Design review of the part built by this model. Coordinates are the model's own, in mm. Face numbers are marked on the shaded views. Round coordinates to 2 decimals unless told otherwise and drop trailing zeros. Order: outer loops, then holes, each group sorted by start corner. A loop starts at its lowest first (then second) coordinate and runs counter-clockwise, first axis right, second up.
from build123d import *

# Parameters (mm, degrees)
BOSS_EXTRUDE1_DEPTH = 6.35
SKETCH2_R           = 1.5875
SKETCH2_W           = 23.495
SKETCH2_H           = 23.495
SKETCH2_R_2         = 8.763
SKETCH2_R_3         = 1.27
SKETCH2_R_4         = 2.159
SKETCH2_R_5         = 2.2225
SKETCH2_R_6         = 31.75
SKETCH2_R_7         = 20.32
SKETCH2_R_8         = 9.525
CUT_EXTRUDE1_DEPTH  = 7.35


with BuildPart() as part:
    # Sketch1 → Boss-Extrude1 (new body)
    with BuildSketch(Plane.XY):
        Polygon((-249.2375, 225.334147625), (249.2375, 225.334147625), (95.25, -225.334147625), (-95.25, -225.334147625), align=None)
    extrude(amount=BOSS_EXTRUDE1_DEPTH)

    # Sketch2 → Cut-Extrude1 (cut, through all)
    with BuildSketch(Plane.XY.offset(6.35)):
        with Locations((-47.625, 15.784147625)):
            Circle(SKETCH2_R)
        with Locations((-47.625, 111.034147625)):
            Circle(SKETCH2_R)
        with Locations((47.625, 15.784147625)):
            Circle(SKETCH2_R)
        with Locations((47.625, 111.034147625)):
            Circle(SKETCH2_R)
        with Locations((0, 174.534147625)):
            Rectangle(SKETCH2_W, SKETCH2_H)
        with Locations((-101.6, 111.034147625)):
            Circle(SKETCH2_R_2)
        with Locations((15, 174.534147625)):
            Circle(SKETCH2_R_3)
        with Locations((-15, 174.534147625)):
            Circle(SKETCH2_R_3)
        with Locations((-40.216666667, -190.409147625)):
            Circle(SKETCH2_R)
        with Locations((-31.75, -203.109147625)):
            Circle(SKETCH2_R)
        with Locations((31.75, -190.409147625)):
            Circle(SKETCH2_R)
        with Locations((40.216666667, -203.109147625)):
            Circle(SKETCH2_R)
        with Locations((-77.7875, -29.409256694)):
            Circle(SKETCH2_R_4)
        with Locations((-23.8125, -29.409256694)):
            Circle(SKETCH2_R_4)
        with Locations((-77.7875, -83.384256694)):
            Circle(SKETCH2_R_4)
        with Locations((-23.8125, -83.384256694)):
            Circle(SKETCH2_R_4)
        with Locations((-83.185, 44.994147625)):
            Circle(SKETCH2_R_5)
        with Locations((-50.8, -56.396756694)):
            Circle(SKETCH2_R_6)
        with Locations((-120.015, 44.994147625)):
            Circle(SKETCH2_R_5)
        with Locations((-120.015, 81.824147625)):
            Circle(SKETCH2_R_5)
        with Locations((-83.185, 81.824147625)):
            Circle(SKETCH2_R_5)
        with Locations((-101.6, 63.409147625)):
            Circle(SKETCH2_R_7)
        with Locations((120.015, 44.994147625)):
            Circle(SKETCH2_R_5)
        with Locations((83.185, 44.994147625)):
            Circle(SKETCH2_R_5)
        with Locations((83.185, 81.824147625)):
            Circle(SKETCH2_R_5)
        with Locations((-83.079166667, 199.934147625)):
            Circle(SKETCH2_R_8)
        with Locations((83.079166667, 199.934147625)):
            Circle(SKETCH2_R_8)
        with Locations((120.015, 81.824147625)):
            Circle(SKETCH2_R_5)
        with Locations((101.6, 63.409147625)):
            Circle(SKETCH2_R_7)
        with Locations((23.8125, -29.409256694)):
            Circle(SKETCH2_R_4)
        with Locations((77.7875, -29.409256694)):
            Circle(SKETCH2_R_4)
        with Locations((23.8125, -83.384256694)):
            Circle(SKETCH2_R_4)
        with Locations((77.7875, -83.384256694)):
            Circle(SKETCH2_R_4)
        with Locations((50.8, -56.396756694)):
            Circle(SKETCH2_R_6)
    extrude(amount=-CUT_EXTRUDE1_DEPTH, mode=Mode.SUBTRACT)


solid = part.part
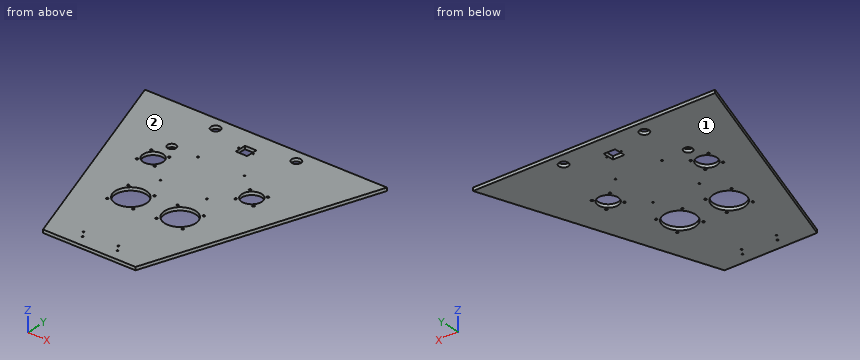
1) Take a section at A-A on y = -64.5. Give the boundary of the cut face in (x, z).
Results:
outline: (-150.2, 0) - (-81.5, 0) - (-81.5, 6.35) - (-150.2, 6.35) - close; (-20.1, 0) - (20.1, 0) - (20.1, 6.35) - (-20.1, 6.35) - close; (81.5, 0) - (150.2, 0) - (150.2, 6.35) - (81.5, 6.35) - close
2) Take a section at B-B on x = 101.6. Give the boundary of the cut face in (y, z).
Results:
outline: (-206.75, 0) - (43.09, 0) - (43.09, 6.35) - (-206.75, 6.35) - close; (83.73, 0) - (225.33, 0) - (225.33, 6.35) - (83.73, 6.35) - close
3) To check wall thickness, follow line 1 along Y through (x, z) = (-0.5, 1); line 2 along X through (y, z) = (14.5, 0.5); line 3 along X through (y, z) = (73.5, 1). State the ranges of each line that lie inside material, in increasing order.
Results:
line 1: y = -225.33 to 162.79, 186.28 to 225.33
line 2: x = -177.2 to -48.56, -46.69 to 46.69, 48.56 to 177.2
line 3: x = -197.36 to -119.24, -83.96 to 83.96, 119.24 to 197.36
4) The part is to be moulded in two halves that separate along Z. For the marked faces 1 and 2, say which applies: released by +Z, released by -Z, zero draft, split by the parting line, or undercut.
Results:
face 1: released by -Z
face 2: released by +Z
5) Take a section at C-C on y = 55. Give the boundary of the cut face in (x, z), plus the area to 3 significant figures.
Results:
outline: (-191.04, 0) - (-120.1, 0) - (-120.1, 6.35) - (-191.04, 6.35) - close; (-83.1, 0) - (83.1, 0) - (83.1, 6.35) - (-83.1, 6.35) - close; (120.1, 0) - (191.04, 0) - (191.04, 6.35) - (120.1, 6.35) - close
area: 1,960 mm2
6) Take a section at D-D on z = 1. State how many separate pieces and enclosed holes the cut face has, plus the area to 3 significant figures.
Results:
separate pieces: 1
enclosed holes: 34
area: 145,000 mm2
